Verification items for the finished model (mm, model axes). A direction names the side the tool comes from. Round coordinates to 2 decimals unless told otherwise and drop trailing zeros. Order: outer loops, then holes, each group sorted by start corner. A loop starts at its lowest first (then second) coordinate and runs counter-clockwise, first axis right, second up. Notation, with made-up numbers: (11.25, 62.25) -> (52.25, 62.25) arc R12 cw to (52.25, 83.25) -> close; hole circle Ø3 at (34, 34). An arc over 180 degrees is marked (long way). Put each result on its own line as item: value.
from build123d import *

# Parameters (mm, degrees)
SKETCH1_R               = 3
SKETCH1_R_2             = 1.25
MAIN_DEPTH              = 3
SKETCH2_R               = 6
SKETCH2_R_2             = 3
LINEARBALLSUPPORT_DEPTH = 7
FILLET1_R               = 2


with BuildPart() as part:
    # Sketch1 → Main (new body)
    with BuildSketch(Plane.XY):
        with BuildLine():
            Line((-9, 10.723805295), (-9, -10.723805295))
            ThreePointArc((-9, -10.723805295), (0, -14), (9, -10.723805295))
            Line((9, -10.723805295), (9, 10.723805295))
            ThreePointArc((9, 10.723805295), (0, 14), (-9, 10.723805295))
        make_face()
        Circle(SKETCH1_R, mode=Mode.SUBTRACT)
        with Locations((-5, 10)):
            Circle(SKETCH1_R_2, mode=Mode.SUBTRACT)
        with Locations((5, 10)):
            Circle(SKETCH1_R_2, mode=Mode.SUBTRACT)
        with Locations((-5, -10)):
            Circle(SKETCH1_R_2, mode=Mode.SUBTRACT)
        with Locations((5, -10)):
            Circle(SKETCH1_R_2, mode=Mode.SUBTRACT)
    extrude(amount=MAIN_DEPTH)

    # Sketch2 → LinearBallSupport (add)
    with BuildSketch(Plane.XY.offset(3)):
        Circle(SKETCH2_R)
        Circle(SKETCH2_R_2, mode=Mode.SUBTRACT)
    extrude(amount=LINEARBALLSUPPORT_DEPTH)

    # Fillet1
    fillet1_edges = [part.edges().sort_by_distance(p)[0] for p in [
        (-6, 0, 3),
    ]]
    fillet(fillet1_edges, radius=FILLET1_R)


solid = part.part
Item 1: Section check A-A on y = 0. Record the boundary of the cut face in (x, z), then the cut area to 3 significant figures.
Check sheet entries:
outline: (-9, 0) -> (-3, 0) -> (-3, 10) -> (-6, 10) -> (-6, 5) arc R2 cw to (-8, 3) -> (-9, 3) -> close; (3, 0) -> (9, 0) -> (9, 3) -> (8, 3) arc R2 cw to (6, 5) -> (6, 10) -> (3, 10) -> close
area: 79.7 mm^2
Item 2: Section check C-C on y = -10. Record the boundary of the cut face in (x, z), then the cut area to 3 significant figures.
Check sheet entries:
outline: (-9, 0) -> (-6.25, 0) -> (-6.25, 3) -> (-9, 3) -> close; (-3.75, 0) -> (3.75, 0) -> (3.75, 3) -> (-3.75, 3) -> close; (6.25, 0) -> (9, 0) -> (9, 3) -> (6.25, 3) -> close
area: 39.0 mm^2
Item 3: Release check for a two-part mould opening along Y. For faces 3 (the cylindrical face through (0, 14, 1)), 4 (the flat face through (9, 0, 1)), 5 (the cylindrical face through (-3, 0, 5)) record: +Y half, -Y half, draft (parallel to the pull), parting line (faces both ways), or undercut.
Check sheet entries:
face 3: +Y half
face 4: draft
face 5: undercut
Item 4: Section check B-B on x = 0. Record the boundary of the cut face in (y, z).
Check sheet entries:
outline: (-14, 0) -> (-3, 0) -> (-3, 10) -> (-6, 10) -> (-6, 5) arc R2 cw to (-8, 3) -> (-14, 3) -> close; (3, 0) -> (14, 0) -> (14, 3) -> (8, 3) arc R2 cw to (6, 5) -> (6, 10) -> (3, 10) -> close
Item 5: Material ranges on L1, parallel to Y at x = -5, z = 1.1; L2, parallel to Z at x = 3.75, y = -11.25; L3, parallel to Y at x = 0, z = 5.5, recorded low to high. Write a range as [from, to].
Check sheet entries:
L1: y = [-13.08, -11.25], [-8.75, 8.75], [11.25, 13.08]
L2: z = [0, 3]
L3: y = [-6, -3], [3, 6]
Item 6: Section check D-D on z = 1. Record the boundary of the cut face in (x, y).
Check sheet entries:
outline: (-9, -10.72) arc R14 ccw to (9, -10.72) -> (9, 10.72) arc R14 ccw to (-9, 10.72) -> close; hole circle Ø2.5 at (-5, -10); hole circle Ø2.5 at (-5, 10); hole circle Ø6 at (0, 0); hole circle Ø2.5 at (5, -10); hole circle Ø2.5 at (5, 10)
Item 7: Tool access check on faces 1 (the cylindrical face through (4.84, -8.76, 1.48)), 2 (the cylindrical face through (-6, 0, 7)). Record the directions out of +Z, -Z, +X, -X, +Y, -Y that give a thin tool (end or side, any length) a straight path to the whole face; none if there is none.
Check sheet entries:
face 1: +Z, -Z
face 2: +Z
Item 8: Gauge pin test, flat ends, axial feed: pin 1 Ø5 at (y, z) = (-9.5, 7.5) entering from +X; pin 2 Ø1.5 at (x, z) = (3.5, 5.5) entering from +Y; pin 3 Ø3 at (x, y) = (5, 10) entering from +Z. Record the tip position at first contact, or that the pin passes through.
Check sheet entries:
pin 1: passes through
pin 2: stops at y = 5.33
pin 3: stops at z = 3
